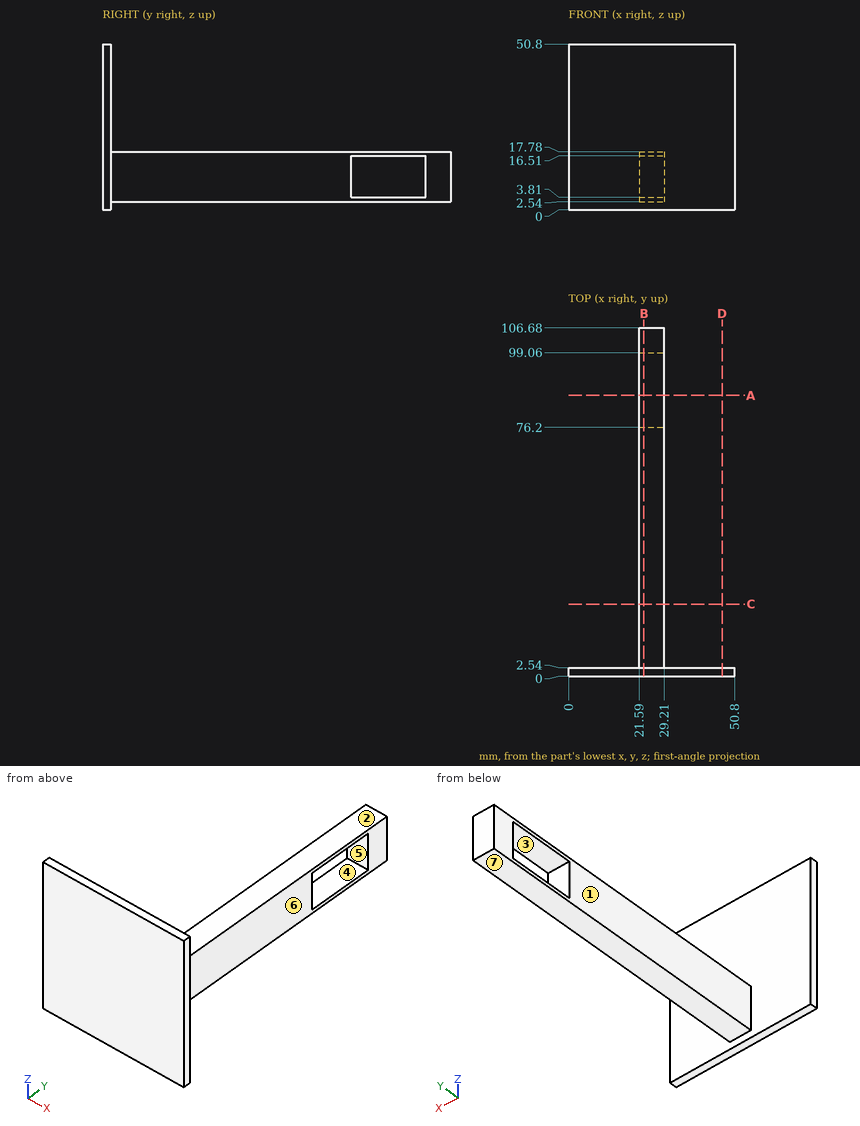
Geometry check sheet. Reference: drawing and pictorial views, mm from the part's lowest x, y, z. A direction names the side the tool comes from. Give positions to 0.01 mm unless a question says otherwise; leave off trailing zeros. Loops run counter-clockwise (first coordinate to the right, second up) from the corner with the lowest first, then second, coordinate; pieces in that order, holes last. Notation, with made-up numbers: (-4, -6) -> (54, -6) arc R24 cw to (54, 11) -> close; hole circle Ø4 at (68, -12). An arc over 180 degrees is marked (long way). Answer in a Markdown table with one row per item. Add a question column.
1) Gauge pin test, flat ends, axial feed: P1, Ø10, axis at x = 19.5, z = 41.5, coming from the -Y side; P2, Ø10, axis at y = 59, z = 16, coming from the -X side; P3, Ø12, axis at x = 28, y = 30, coming from the +Z side; P4, Ø8, axis at x = 29, y = 36.5, coming from the -Z side. Record the tip position at first contact, or that the pin passes through.
2) Draft check along Z on the marked faces 1, 2, 3 and 4. Enter one of: pulls with the +Z half, pulls with the -Z half, needs draft (parallel to the pull), parting line crosses it, or undercut.
3) Cross-section at B-B on x = 23. Record the boundary of the cut face in (y, z), and give its area (3 significant figures).
4) Cross-section at C-C on y = 22. Record the boundary of the cut face in (x, z).
5) Cross-section at A-A on y = 86. Record the boundary of the cut face in (x, z).
6) Material ranges on probe 1 along Z at (x, y) = (23, 88.5); probe 2 along X at (y, z) = (23.5, 16); probe 3 along Y at (x, z) = (7, 10.5), recorded low to high. Write a range as from..to.
7) Cross-section at D-D on x = 47. Record the boundary of the cut face in (y, z).
8) Set-up check for the marked faces 5, 6 and 7: record each of +Z, -Z, +X, -X, +Y, -Y from which the full face is reachable in a straight line by a thin tool's end or side.
Outcome:
| question | item | result |
|---|---|---|
| 1 | P1 | stops at y = 0 |
| 1 | P2 | stops at x = 21.59 |
| 1 | P3 | stops at z = 17.78 |
| 1 | P4 | stops at z = 2.54 |
| 2 | face 1 | needs draft |
| 2 | face 2 | pulls with the +Z half |
| 2 | face 3 | undercut |
| 2 | face 4 | undercut |
| 3 | outline | (0, 0) -> (2.54, 0) -> (2.54, 2.54) -> (106.68, 2.54) -> (106.68, 17.78) -> (2.54, 17.78) -> (2.54, 50.8) -> (0, 50.8) -> close; hole (76.2, 3.81) -> (99.06, 3.81) -> (99.06, 16.51) -> (76.2, 16.51) -> close |
| 3 | area | 1,430 mm^2 |
| 4 | outline | (21.59, 2.54) -> (29.21, 2.54) -> (29.21, 17.78) -> (21.59, 17.78) -> close |
| 5 | outline | (21.59, 2.54) -> (29.21, 2.54) -> (29.21, 3.81) -> (21.59, 3.81) -> close; (21.59, 16.51) -> (29.21, 16.51) -> (29.21, 17.78) -> (21.59, 17.78) -> close |
| 6 | probe 1 | z = 2.54..3.81, 16.51..17.78 |
| 6 | probe 2 | x = 21.59..29.21 |
| 6 | probe 3 | y = 0..2.54 |
| 7 | outline | (0, 0) -> (2.54, 0) -> (2.54, 50.8) -> (0, 50.8) -> close |
| 8 | face 5 | +X, -X |
| 8 | face 6 | +Z, -Z, +X, +Y |
| 8 | face 7 | -Z, +X, -X, +Y |
